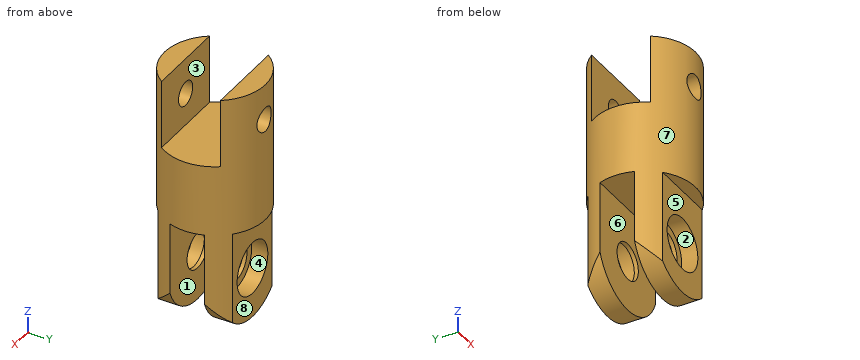
```python
from build123d import *

# Parameters (mm, degrees)
SKETCH_1_R               = 12.5
EXTRUDE_1_DEPTH          = 60.686921397
CUT_EXTRUDE_START        = -26
CUT_EXTRUDE_1_DEPTH      = 26
SKETCH_3_R               = 4.5
CUT_EXTRUDE_2_DEPTH      = 34.123937734
SKETCH_6_R               = 6.5
CUT_EXTRUDE_5_DEPTH      = 4
CUT_EXTRUDE_6_DEPTH      = 17
CUT_EXTRUDE_7_DEPTH      = 29
CUT_EXTRUDE_7_DEPTH_BACK = 17
SKETCH_9_R               = 3


with BuildPart() as part:
    # 스케치1 → 보스-돌출1 (new body)
    with BuildSketch(Plane.XY):
        Circle(SKETCH_1_R)
    extrude(amount=-EXTRUDE_1_DEPTH)

    # 스케치2 → 컷-돌출1 (cut)
    with BuildSketch(Plane(origin=(0, 0, -60.686921397), x_dir=(-1, 0, 0), z_dir=(0, 0, -1)).offset(CUT_EXTRUDE_START)):
        with BuildLine():
            Line((8.371418841, 9.282744561), (-8.371418841, 9.282744561))
            ThreePointArc((-8.371418841, 9.282744561), (0, 12.5), (8.371418841, 9.282744561))
        make_face()
        with BuildLine():
            Line((11.743427908, 4.282744561), (-11.743427908, 4.282744561))
            ThreePointArc((-11.743427908, 4.282744561), (-12.5, 0), (-11.743427908, -4.282744561))
            Line((-11.743427908, -4.282744561), (11.743427908, -4.282744561))
            ThreePointArc((11.743427908, -4.282744561), (12.5, 0), (11.743427908, 4.282744561))
        make_face()
        with BuildLine():
            Line((8.371418841, -9.282744561), (-8.371418841, -9.282744561))
            ThreePointArc((-8.371418841, -9.282744561), (0, -12.5), (8.371418841, -9.282744561))
        make_face()
    extrude(amount=CUT_EXTRUDE_1_DEPTH, mode=Mode.SUBTRACT)

    # 스케치3 → 컷-돌출2 (cut)
    with BuildSketch(Plane(origin=(0, 9.282744561, 0), x_dir=(1, 0, 0), z_dir=(0, 1, 0))):
        with Locations(Location((0, 48.186921397, 0), (0, 0, 270))):
            Circle(SKETCH_3_R)
        with BuildLine():
            Line((-22.5, 48.186921397), (-12.5, 48.186921397))
            ThreePointArc((-12.5, 48.186921397), (0, 60.686921397), (12.5, 48.186921397))
            Line((12.5, 48.186921397), (22.5, 48.186921397))
            ThreePointArc((22.5, 48.186921397), (0, 70.686921397), (-22.5, 48.186921397))
        make_face()
    extrude(amount=-CUT_EXTRUDE_2_DEPTH, mode=Mode.SUBTRACT)

    # 스케치6 → 컷-돌출5 (cut)
    with BuildSketch(Plane(origin=(0, 9.282744561, 0), x_dir=(1, 0, 0), z_dir=(0, 1, 0))):
        with Locations(Location((0, 48.186921397, 0), (0, 0, 270))):
            Circle(SKETCH_6_R)
    cut_extrude_5 = extrude(amount=-CUT_EXTRUDE_5_DEPTH, mode=Mode.SUBTRACT)

    # 대칭 복사3: 컷-돌출5 across plane
    add(cut_extrude_5.mirror(Plane.ZX), mode=Mode.SUBTRACT)

    # 스케치8 → 컷-돌출6 (cut)
    with BuildSketch(Plane.XY):
        with BuildLine():
            Line((10.159210883, 7.282886395), (-10.159210883, 7.282886395))
            ThreePointArc((-10.159210883, 7.282886395), (-12.5, 0), (-10.159210883, -7.282886395))
            Line((-10.159210883, -7.282886395), (10.159210883, -7.282886395))
            ThreePointArc((10.159210883, -7.282886395), (12.5, 0), (10.159210883, 7.282886395))
        make_face()
    extrude(amount=-CUT_EXTRUDE_6_DEPTH, mode=Mode.SUBTRACT)

    # 스케치9 → 컷-돌출7 (cut, two sides: drawn at the far end of the back side and taken through both)
    with BuildSketch(Plane(origin=(0, -7.282886395, 0), x_dir=(1, 0, 0), z_dir=(0, 1, 0)).offset(-CUT_EXTRUDE_7_DEPTH_BACK)):
        with Locations(Location((0, 8.940465454, 0), (0, 0, 90))):
            Circle(SKETCH_9_R)
    extrude(amount=CUT_EXTRUDE_7_DEPTH + CUT_EXTRUDE_7_DEPTH_BACK, mode=Mode.SUBTRACT)


solid = part.part
```
Could you check a few things on this model? Use its own coordinates, in mm. Face numbers are marked on the shaded views. A direction names the side the tool comes from. Round coordinates to 2 decimals unless told otherwise and drop trailing zeros. Write each loop counter-clockwise with the first axis right and the second up, starting at its lowest first coordinate (ties: lowest second). Pieces come first, ordered by that corner, then holes. Notation, with made-up numbers: M 65.25,63.25 L 116.25,63.25 A20 ccw 116.25,80.25 Z; hole C 32,23.5 d2. An arc over 180 degrees is marked long. Write each question's results on one line, items separated by ' | '. Start each with the question number.
1. Imagine slicing it at B-B on x = 0. Count the separate pieces of the cut face and the enclosed holes in it, and give its area (3 significant figures).
2. On a 3-axis mill with a long thin cutter (end or side, diameter ignored), from which of +Z, -Z, +X, -X, +Y, -Y can I reach the whole of each face in a straight line? I mean the marked faces 1, 2, 3, 4 and 5. Say none if no direction works.
3. I need wall thicknesses on L1, parallel to Y at x = 7.5, z = -50.5; L2, parallel to Y at x = 5.75, z = -49; L3, parallel to Z at x = -1.25, y = 3.5. Which ranges of each line are inside material? Lowest first, please. Write a range as from..to.
4. Thinking about a two-plate mould opening in Y: for the marked faces 6, 7 and 8, which applies, +Y half, -Y half, draft (parallel to the pull), parting line (faces both ways), or undercut?
5. Imagine slicing it at A-A on z = -39. List the corners of the cut face in (x, y) for me.
6. Imagine slicing it at D-D on x = -7.25. List the corners of the cut face in (y, z) for me, and give its area (3 significant figures).
7. I'm going to push flat-ended pins straight in: pin 1 Ø7.5 at (x, y) = (3, -2) entering from +Z; pin 2 Ø5 at (x, y) = (3, 5) entering from -Z; pin 3 Ø10 at (y, z) = (6, -15) entering from +X. Where does each tip first touch, or does it pass through?
8. Imagine slicing it at C-C on y = -6.5. List the corners of the cut face in (x, z) for me.
Result sheet:
1) separate pieces: 5 | enclosed holes: 0 | area: 695 mm^2
2) face 1: -Z, +X, -X | face 2: -Y | face 3: +Z, +X, -X | face 4: +Y | face 5: -Z, +X, -X, -Y
3) L1: y = -9.28..-4.28, 4.28..9.28 | L2: y = -5.28..-4.28, 4.28..5.28 | L3: z = -34.69..-17
4) face 6: undercut | face 7: parting line | face 8: +Y half
5) outline: M -11.74,-4.28 A12.5 ccw -8.37,-9.28 L 8.37,-9.28 A12.5 ccw 11.74,-4.28 Z; M -11.74,4.28 L 11.74,4.28 A12.5 ccw 8.37,9.28 L -8.37,9.28 A12.5 ccw Z
6) outline: M -10.18,-34.69 L -9.28,-34.69 L -9.28,-58.37 L -4.28,-58.37 L -4.28,-34.69 L 4.28,-34.69 L 4.28,-58.37 L 9.28,-58.37 L 9.28,-34.69 L 10.18,-34.69 L 10.18,0 L 7.28,0 L 7.28,-17 L -7.28,-17 L -7.28,0 L -10.18,0 Z | area: 696 mm^2
7) pin 1: stops at z = -17 | pin 2: stops at z = -60.68 | pin 3: stops at x = 12.42
8) outline: M -10.68,-54.69 A12.5 ccw 10.68,-54.69 L 10.68,-17 L -10.68,-17 Z; hole C 0,-48.19 d13
